from build123d import *


with BuildPart() as f1:
    # F0 (on Top) → F1 (revolve)
    with BuildSketch(Plane.XY):
        with BuildLine():
            Line((13.1365, 12.665), (17.399, 12.665))
            Line((17.399, 12.665), (17.399, 14.165))
            Line((17.399, 14.165), (11.1365, 14.165))
            Line((11.1365, 14.165), (11.1365, -14.156))
            Line((11.1365, -14.156), (17.399, -14.156))
            Line((17.399, -14.156), (17.399, -12.656))
            Line((17.399, -12.656), (13.1365, -12.656))
            ThreePointArc((13.1365, -12.656), (12.782947, -12.509553), (12.6365, -12.156))
            Line((12.6365, -12.156), (12.6365, 12.165))
            ThreePointArc((12.6365, 12.165), (12.782947, 12.518553), (13.1365, 12.665))
        make_face()
    revolve(axis=Axis((0, 2.854013, 0), (0, 1, 0)))


solid = f1.part
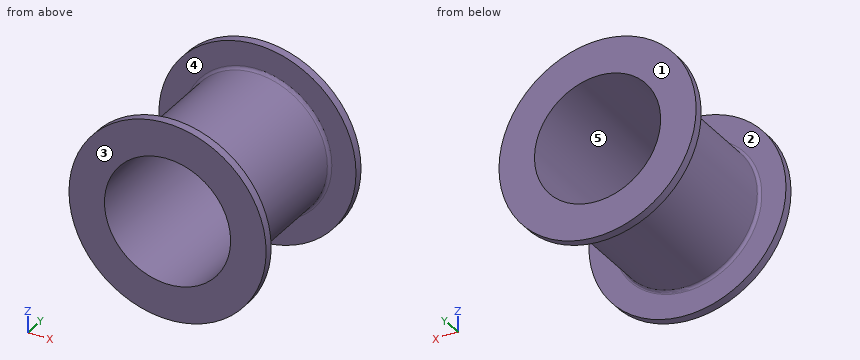
Design review of the part built by this model. Coordinates are the model's own, in mm. Face numbers are marked on the shaded views. A direction names the side the tool comes from. Give positions to 0.01 mm unless a question says otherwise; leave off trailing zeros. Order: outer loops, then holes, each group sorted by start corner. A loop starts at its lowest first (then second) coordinate and runs counter-clockwise, first axis right, second up.
1. Add section B-B, the plane y = 6. State the section outline as (x, z) points.
Solution:
outline: circle Ø25.27 at (0, 0); hole circle Ø22.27 at (0, 0)
2. Tool access review of the marked faces 4 and 5: name each direction out of +Z, -Z, +X, -X, +Y, -Y from which nothing blocks a thin tool from reaching the whole face with its end or side.
Solution:
face 4: none
face 5: +Y, -Y
3. Add section A-A, the plane x = 0. State the section outline as (y, z) points (1 decimal).
Solution:
outline: (-14.2, -17.4) - (-12.7, -17.4) - (-12.7, -13.1) arc R0.5 cw to (-12.2, -12.6) - (12.2, -12.6) arc R0.5 cw to (12.7, -13.1) - (12.7, -17.4) - (14.2, -17.4) - (14.2, -11.1) - (-14.2, -11.1) - close; (-14.2, 11.1) - (14.2, 11.1) - (14.2, 17.4) - (12.7, 17.4) - (12.7, 13.1) arc R0.5 cw to (12.2, 12.6) - (-12.2, 12.6) arc R0.5 cw to (-12.7, 13.1) - (-12.7, 17.4) - (-14.2, 17.4) - close
4. For pin 1 Ø5 at (y, z) = (9.5, 8.5) entering from -X; pin 2 Ø13.5 at (x, z) = (0, 0) entering from -Y; pin 3 Ø4 at (x, y) = (-8, -10.5) entering from +Z; pin 4 Ø5 at (x, y) = (-2.5, -4) entering from +Z, all flat-tipped, find the tip position at first contact; note any pin that passes through.
Solution:
pin 1: stops at x = -11.12
pin 2: passes through
pin 3: stops at z = 11.12
pin 4: stops at z = 12.64
5. Mouldability with a two-part tool opening along Y and no side actions: class the marked faces 1, 2 and 3 as +Y half, -Y half, draft (parallel to the pull), parting line (faces both ways), or undercut.
Solution:
face 1: +Y half
face 2: undercut
face 3: -Y half
6. To check wall thickness, follow L1, parallel to X at y = -7, z = 0; L2, parallel to Y at x = -3.5, z = -15.5 (3 decimals). State the ranges of each line that lie inside material, in increasing order.
Solution:
L1: x = -12.64 to -11.14, 11.14 to 12.64
L2: y = -14.156 to -12.656, 12.665 to 14.165
